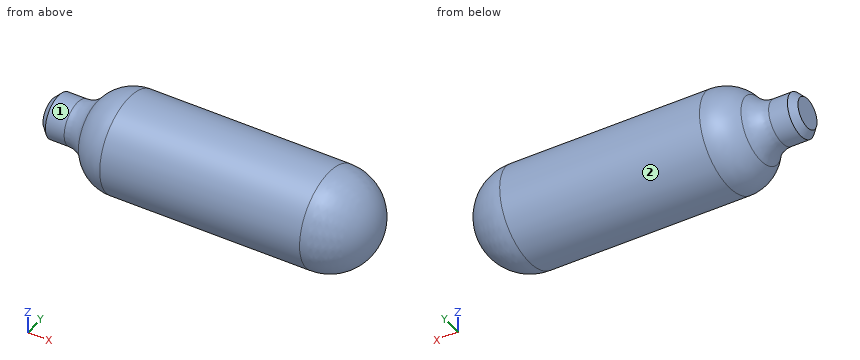
```python
from build123d import *

# Parameters (mm, degrees)
F3_R    = 5.08
F4_SIZE = 1.27


# Not quite as in the source:
# - a fillet or chamfer that OpenCascade refuses, or shapes differently, is made with other operations: its cross-section is extruded or revolved along the edge and cut away or added


with BuildPart() as f1:
    # F0 (on Front) → F1 (revolve)
    with BuildSketch(Plane.XZ):
        with BuildLine():
            Line((-65.912999015, 22.4110006839), (-65.912999015, 18.1610006839))
            Line((-65.912999015, 18.1610006839), (-1.912999015, 18.1610006839))
            Line((-1.912999015, 18.1610006839), (-1.912999015, 18.1654242131))
            ThreePointArc((-1.912999015, 18.1654242131), (-4.6948756483, 24.8821639675), (-11.4112079773, 27.6650241112))
            Line((-11.4112079773, 27.6650241112), (-57.911999015, 27.6650241112))
            Line((-57.911999015, 27.6650241112), (-57.911999015, 22.4110006839))
            Line((-57.911999015, 22.4110006839), (-65.912999015, 22.4110006839))
        make_face()
    revolve(axis=Axis((-33.912999015, 0, 18.1610006839), (1, 0, 0)))

    # F2: fillet of radius 7.62 on 1 edges, made by hand

    # F2_s1 → F2_t2 (revolve, cut)
    with BuildSketch(Plane.XZ):
        with BuildLine():
            ThreePointArc((-50.6686189437, 27.6650241112), (-55.1427478263, 26.2132143435), (-57.911999015, 22.4110006839))
            Line((-57.911999015, 22.4110006839), (-57.911999015, 27.6650241112))
            Line((-57.911999015, 27.6650241112), (-50.6686189437, 27.6650241112))
        make_face()
    revolve(axis=Axis((-57.911999015, 0, 18.1610006839), (1, 0, 0)), mode=Mode.SUBTRACT)

    # F3
    f3_edges = [f1.edges().sort_by_distance(p)[0] for p in [
        (-57.911999, 0, 13.911001),
    ]]
    fillet(f3_edges, radius=F3_R)

    # F4
    f4_edges = [f1.edges().sort_by_distance(p)[0] for p in [
        (-65.912999, 0, 13.911001),
    ]]
    chamfer(f4_edges, length=F4_SIZE)


solid = f1.part
```
Could you check a few things on this model? Use its own coordinates, in mm. Face numbers are marked on the shaded views. A direction names the side the tool comes from. Coordinates: 2 decimals unless noted, no trailing zeros. Write each loop counter-clockwise with the first axis right and the second up, starting at its lowest first coordinate (ties: lowest second). Pieces come first, ordered by that corner, then holes. Notation, with made-up numbers: (18, -36.75) -> (50, -36.75) arc R13 cw to (50, -13.75) -> close; hole circle Ø9 at (80, 19). An arc over 180 degrees is marked (long way). Return JSON: item names as keys, results as strings.
(1) I need wall thicknesses on L1, parallel to X at y = -3.25, z = 17.75; L2, parallel to Y at x = -43, z = 23; L3, parallel to X at y = 6.5, z = 15. Which ranges of each line are inside material? Lowest first, please.
Numbers:
{"L1": "x = -65.62 to -2.49", "L2": "y = -8.18 to 8.18", "L3": "x = -56.1 to -5.24"}
(2) I'm going to push flat-ended pins straight in: pin 1 (2 mm diameter, centred on x = -46.5, y = -5, fed in from -Z); pin 2 (6 mm diameter, centred on y = -5.5, z = 12, fed in from +X); pin 3 (2 mm diameter, centred on y = 3.5, z = 14.5, fed in from +X). Where does each tip first touch, or does it pass through?
Numbers:
{"pin 1": "stops at z = 9.54", "pin 2": "stops at x = -3.5", "pin 3": "stops at x = -2.82"}
(3) Which directions (+Z, -Z, +X, -X, +Y, -Y) give clear straight access to the entire face, cutting with the end or side of a thin tool? Please do the marked faces 1 and 2.
Numbers:
{"face 1": "-X", "face 2": "+X, -X"}
(4) Imagine slicing it at A-A, the plane x = -47. Please give me the cut outline in (y, z).
Numbers:
{"outline": "circle Ø19.01 at (0, 18.16)"}
